from build123d import *

# Parameters (mm, degrees)
BOSS_EXTRUDE1_DEPTH            = 8
CBORE_FOR_M5_SHCS1_AT_2_COUNT  = 2
CBORE_FOR_M5_SHCS1_AT_2_PITCH  = 20
SKETCH5_W                      = 25
SKETCH5_H                      = 2.975
BOSS_EXTRUDE2_DEPTH            = 12.51
SKETCH6_W                      = 3
SKETCH6_H                      = 8.01
BOSS_EXTRUDE3_DEPTH            = 7.5
BOSS_EXTRUDE4_DEPTH            = 5.5
SKETCH8_W                      = 17
SKETCH8_H                      = 1.25
BOSS_EXTRUDE5_DEPTH            = 7.5
BOSS_EXTRUDE6_DEPTH            = 5.4
FILLET2_R                      = 1
CBORE_FOR_M3_SHCS1_D           = 3.6
CBORE_FOR_M3_SHCS1_DEPTH       = 5
CBORE_FOR_M3_SHCS1_CBORE_D     = 6.5
CBORE_FOR_M3_SHCS1_CBORE_DEPTH = 3
SKETCH13_R                     = 2.4
CUT_EXTRUDE1_DEPTH             = 3.8
SKETCH14_R                     = 1.65
CUT_EXTRUDE2_DEPTH             = 3
SKETCH15_W                     = 20
SKETCH15_H                     = 20
CUT_EXTRUDE3_DEPTH             = 29
SKETCH16_W                     = 17
SKETCH16_H                     = 0.2
SKETCH16_W_2                   = 3
SKETCH16_H_2                   = 0.3
CUT_EXTRUDE4_DEPTH             = 7.5


with BuildPart() as part:
    # Sketch1 → Boss-Extrude1 (new body)
    with BuildSketch(Plane(origin=(0, 0, 0), x_dir=(1, 0, 0), z_dir=(0, 1, 0))):
        Polygon((-10, 0), (-15, 0), (-15, 20), (-10, 20), (10, 20), (10, -20), (-10, -20), align=None)
    extrude(amount=BOSS_EXTRUDE1_DEPTH)

    # Sketch4 → CBORE for M5 SHCS1 (revolve, cut)
    with BuildSketch(Plane(origin=(0, 8, -10), x_dir=(0, 0, 1), z_dir=(1, 0, 0))):
        Polygon((0, 0), (0, 8), (2.75, 8), (2.75, 5), (5, 5), (5, 0.025), (5.025, 0), align=None)
    cbore_for_m5_shcs1 = revolve(axis=Axis((0, 14.35, -10), (0, -1, 0)), mode=Mode.SUBTRACT)

    # CBORE for M5 SHCS1 at 2: CBORE for M5 SHCS1 ×2
    with Locations(*[(0, 0, i * CBORE_FOR_M5_SHCS1_AT_2_PITCH) for i in range(1, CBORE_FOR_M5_SHCS1_AT_2_COUNT)]):
        add(cbore_for_m5_shcs1, mode=Mode.SUBTRACT)

    # Sketch5 → Boss-Extrude2 (add)
    with BuildSketch(Plane(origin=(0, 8, 0), x_dir=(1, 0, 0), z_dir=(0, 1, 0))):
        with Locations((-2.5, 16.5125)):
            Rectangle(SKETCH5_W, SKETCH5_H)
    extrude(amount=BOSS_EXTRUDE2_DEPTH)

    # Sketch6 → Boss-Extrude3 (add)
    with BuildSketch(Plane(origin=(0, 0, -18), x_dir=(-1, 0, 0), z_dir=(0, 0, -1))):
        Polygon((-10, 20.51), (15, 20.51), (15, 17.51), (-5, 17.51), (-5, 8), (-10, 8), (-10, 20), align=None)
        with Locations((13.5, 12.005)):
            Rectangle(SKETCH6_W, SKETCH6_H)
    extrude(amount=BOSS_EXTRUDE3_DEPTH)

    # Sketch7 → Boss-Extrude4 (add)
    with BuildSketch(Plane(origin=(0, 0, -20), x_dir=(-1, 0, 0), z_dir=(0, 0, -1))):
        Polygon((-10, 0), (15, 0), (15, 8), (12, 8), (-5, 8), (-10, 8), align=None)
    extrude(amount=BOSS_EXTRUDE4_DEPTH)

    # Sketch8 → Boss-Extrude5 (add)
    with BuildSketch(Plane(origin=(0, 0, -18), x_dir=(-1, 0, 0), z_dir=(0, 0, -1))):
        with Locations((3.5, 8.625)):
            Rectangle(SKETCH8_W, SKETCH8_H)
    extrude(amount=BOSS_EXTRUDE5_DEPTH)

    # Sketch9 → Boss-Extrude6 (add)
    with BuildSketch(Plane(origin=(0, 0, -25.5), x_dir=(-1, 0, 0), z_dir=(0, 0, -1))):
        Polygon((-10, 0), (15, 0), (15, -5.4), (9.9, -5.4), (9.9, -20), (-10, -20), align=None)
    extrude(amount=-BOSS_EXTRUDE6_DEPTH)

    # Fillet2
    fillet2_edges = [part.edges().sort_by_distance(p)[0] for p in [
        (10, 0, -0.05),
        (-15, 0, -10.05),
        (10, -20, -22.8),
        (-15, -5.4, -22.8),
        (-9.9, -20, -22.8),
        (-10, 8, 10),
        (-15, 8, -7.5125),
        (-15, 20.51, -20.2625),
        (10, 20.51, -20.2625),
        (10, 8, 2.4875),
    ]]
    fillet(fillet2_edges, radius=FILLET2_R)

    # CBORE for M3 SHCS1
    with Locations(Plane(origin=(10, 0, 0), x_dir=(0, 0, -1), z_dir=(1, 0, 0))):
        with Locations((21.5, 12.48)):
            CounterBoreHole(CBORE_FOR_M3_SHCS1_D / 2, CBORE_FOR_M3_SHCS1_CBORE_D / 2, CBORE_FOR_M3_SHCS1_CBORE_DEPTH, depth=CBORE_FOR_M3_SHCS1_DEPTH)

    # Sketch13 → Cut-Extrude1 (cut)
    with BuildSketch(Plane(origin=(0, 0, -25.5), x_dir=(-1, 0, 0), z_dir=(0, 0, -1))):
        with Locations((10, 4)):
            Circle(SKETCH13_R)
        with Locations((-5, 4)):
            Circle(SKETCH13_R)
    extrude(amount=-CUT_EXTRUDE1_DEPTH, mode=Mode.SUBTRACT)

    # Sketch14 → Cut-Extrude2 (cut)
    with BuildSketch(Plane(origin=(0, 0, -21.7), x_dir=(-1, 0, 0), z_dir=(0, 0, -1))):
        with Locations((-5, 4)):
            Circle(SKETCH14_R)
        with Locations((10, 4)):
            Circle(SKETCH14_R)
    extrude(amount=-CUT_EXTRUDE2_DEPTH, mode=Mode.SUBTRACT)

    # Sketch15 → Cut-Extrude3 (cut, through all)
    with BuildSketch(Plane(origin=(0, 8, 0), x_dir=(1, 0, 0), z_dir=(0, 1, 0))):
        with Locations((0, -10)):
            Rectangle(SKETCH15_W, SKETCH15_H)
    extrude(amount=-CUT_EXTRUDE3_DEPTH, mode=Mode.SUBTRACT)

    # Sketch16 → Cut-Extrude4 (cut)
    with BuildSketch(Plane(origin=(0, 0, -25.5), x_dir=(-1, 0, 0), z_dir=(0, 0, -1))):
        with Locations((3.5, 9.15)):
            Rectangle(SKETCH16_W, SKETCH16_H)
        with Locations((13.5, 15.86)):
            Rectangle(SKETCH16_W_2, SKETCH16_H_2)
    extrude(amount=-CUT_EXTRUDE4_DEPTH, mode=Mode.SUBTRACT)


solid = part.part
Build history of the part. All positions in model axes, mm. A direction names the side the tool comes from. Coordinates: 2 decimals unless noted, no trailing zeros. Write each loop counter-clockwise with the first axis right and the second up, starting at its lowest first coordinate (ties: lowest second). Pieces come first, ordered by that corner, then holes.
(1) Cut at A-A on y = 12.48. List the corners of the cut face in (x, z) (3 decimals), and give its area (3 significant figures).
(2) Cut at D-D on z = -4. List the corners of the cut face in (x, y).
(3) Cut at C-C on y = 4. List the corners of the cut face in (x, z), and give its area (3 significant figures).
(4) Mould opens along Z. For faces 6 (the flat face through (-15, 8, -19)), 7 (the flat face through (-10, 4, -18.7)), 8 (the flat face through (2.2, 3, -12.2)) say: pulls with the +Z half, pulls with the -Z half, needs draft (parallel to the pull), parting line crosses it, or undercut.
(5) Drill centre lines: line 1 (Y direction, x = -10, z = -24.05); line 2 (X direction, y = 2.1, z = -10); line 3 (Y direction, x = 5.75, z = -20). Where is each one in solid material? Low to high.
(6) Pin check, flat tips, straight feed: pin 1 Ø7 at (x, y) = (1.5, 16.5) entering from +Z (3 decimals); pin 2 Ø12 at (x, z) = (-2.5, -12.5) entering from +Y; pin 3 Ø3 at (y, z) = (12.5, -20) entering from +X; pin 4 Ø6 at (x, z) = (5, -3.5) entering from +Y. Stop position of each tip, or through.
(7) 3-axis set-ups, long thin cutter, end or side, ignore diameter. For faces 1 (the flat face through (-13, 15.71, -22)), 2 (the flat face through (-2.3, 0, -7.7)), 3 (the cylindrical face through (8.521, 10.502, -18.921)), 4 (the cylindrical face through (6.31, 3, -20.22)), 5 (the cylindrical face through (9.715, 7.699, -7.407)): which of +Z, -Z, +X, -X, +Y, -Y reach the whole face in a straight line?
(8) Cut at B-B on z = -10. List the corners of the cut face in (x, y) (3 decimals), and give its area (3 significant figures).
Working result:
1. outline: (-15, -25.5) - (-12, -25.5) - (-12, -18) - (5, -18) - (5, -19.7) - (7, -19.7) - (7, -18.25) - (10, -18.25) - (10, -15.025) - (-15, -15.025) - close; (5, -25.5) - (10, -25.5) - (10, -24.75) - (7, -24.75) - (7, -23.3) - (5, -23.3) - close
1. area: 108 mm2
2. outline: (-15, 1) arc R1 ccw to (-14, 0) - (9, 0) arc R1 ccw to (10, 1) - (10, 7) arc R1 ccw to (9, 8) - (-14, 8) arc R1 ccw to (-15, 7) - close
3. outline: (-15, -25.5) - (-12.4, -25.5) - (-12.4, -21.7) - (-11.65, -21.7) - (-11.65, -18.7) - (-8.35, -18.7) - (-8.35, -21.7) - (-7.6, -21.7) - (-7.6, -25.5) - (2.6, -25.5) - (2.6, -21.7) - (3.35, -21.7) - (3.35, -18.7) - (6.65, -18.7) - (6.65, -21.7) - (7.4, -21.7) - (7.4, -25.5) - (10, -25.5) - (10, 0) - (-15, 0) - close; hole circle Ø10 at (0, -10)
3. area: 503 mm2
4. face 6: needs draft
4. face 7: pulls with the -Z half
4. face 8: undercut
5. line 1: y = -5.4 to 1.6, 6.4 to 9.05, 17.51 to 20.51
5. line 2: x = -15 to -2.75, 2.75 to 10
5. line 3: y = 0 to 2.53, 5.47 to 11.49, 13.47 to 20.51
6. pin 1: stops at z = -15.025
6. pin 2: stops at y = 20.51
6. pin 3: stops at x = 7
6. pin 4: stops at y = 8
7. face 1: -Z, -X
7. face 2: +Z, +X, -X, -Y
7. face 3: +X
7. face 4: -Z
7. face 5: +Z, +X, +Y
8. outline: (-15, 1) arc R1 ccw to (-14, 0) - (-2.75, 0) - (-2.75, 3) - (-5, 3) - (-5, 7.975) - (-5.025, 8) - (-14, 8) arc R1 ccw to (-15, 7) - close; (2.75, 0) - (9, 0) arc R1 ccw to (10, 1) - (10, 7) arc R1 ccw to (9, 8) - (5.025, 8) - (5, 7.975) - (5, 3) - (2.75, 3) - close
8. area: 133 mm2
